Answer from the drawing. Dimensions are ordinates in mm from the lowest x, y and z of the part. A direction names the side the tool comes from. Coordinates: 2 decimals unless noted, no trailing zeros. Write each loop counter-clockwise with the first axis right and the second up, starting at its lowest first coordinate (ties: lowest second). Pieces come first, ordered by that corner, then holes. Notation, with made-up numbers: (71, 2) -> (105, 2) arc R15 ccw to (105, 30) -> close; hole circle Ø3 at (89, 72.25). An arc over 180 degrees is marked (long way). One line per item, written item: value. Start each with the question number.
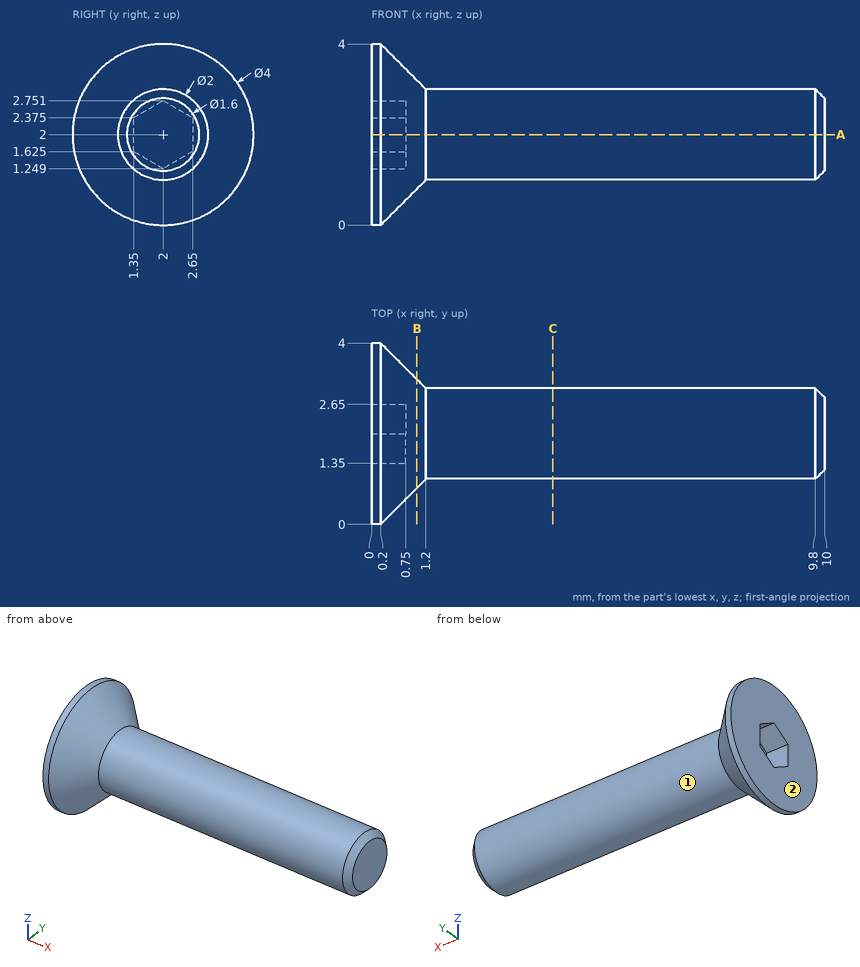
1. A cutting plane is placed at A-A on z = 2. Give the vertices of the cut face in (x, y).
2. A cutting plane is placed at B-B on x = 1. Give the vertices of the cut face in (y, z).
3. Given pin 1 (1 mm diameter, centred on x = 5.5, z = 2, fed in from +Y); pin 2 (1.5 mm diameter, centred on x = 2, y = 2.5, fed in from +Z), each flat-ended and moving along its own axis, determine where each tip first touches the part or whether it passes through.
4. Find the intervals of material crossed by probe 1 along X at (y, z) = (2.4, 2.35); probe 2 along X at (y, z) = (2.4, 2.8) (1 decimal); probe 3 along Y at (x, z) = (8, 2.1) (1 decimal), in increasing order. Write a range as from..to.
5. A tool of negligible diameter and unlimited length cuts with its end or side. For the marked faces 1 and 2, from which of +Z, -Z, +X, -X, +Y, -Y can it reach the whole face along a straight path? Write none if from no direction.
6. A cutting plane is placed at C-C on x = 4. Give the vertices of the cut face in (y, z).
Derived:
1. outline: (0, 0) -> (0.2, 0) -> (1.2, 1) -> (9.8, 1) -> (10, 1.2) -> (10, 2.8) -> (9.8, 3) -> (1.2, 3) -> (0.2, 4) -> (0, 4) -> (0, 2.65) -> (0.75, 2.65) -> (0.75, 1.35) -> (0, 1.35) -> close
2. outline: circle Ø2.4 at (2, 2)
3. pin 1: stops at y = 3
3. pin 2: stops at z = 3
4. probe 1: x = 0.75..10
4. probe 2: x = 0..9.9
4. probe 3: y = 1..3
5. face 1: +X
5. face 2: +Z, -Z, -X, +Y, -Y
6. outline: circle Ø2 at (2, 2)
